Read the model definition and answer for the solid it produces. Units are mm, in the model's axes. A direction names the side the tool comes from. Coordinates: 2 decimals unless noted, no trailing zeros. Loops run counter-clockwise (first coordinate to the right, second up) from the corner with the lowest first, then second, coordinate; pieces in that order, holes last. Notation, with made-up numbers: (-33.5, -35) - (-21.5, -35) arc R30 cw to (-21.5, -8) - close; hole circle Ø1 at (-4.75, -17). An arc over 180 degrees is marked (long way). Use CSV: the item, a comma, the result in double quotes.
```python
from build123d import *

# Parameters (mm, degrees)
SKETCH1_R           = 30
BOSS_EXTRUDE1_DEPTH = 13
SKETCH2_R           = 32.5
BOSS_EXTRUDE2_DEPTH = 1
SKETCH3_R           = 1.6
CUT_EXTRUDE1_DEPTH  = 3.5
SKETCH4_R           = 14
CUT_EXTRUDE2_DEPTH  = 51
SKETCH5_R           = 2.6
CUT_EXTRUDE3_DEPTH  = 25


with BuildPart() as part:
    # Sketch1 → Boss-Extrude1 (new body)
    with BuildSketch(Plane(origin=(0, 0, 0), x_dir=(1, 0, 0), z_dir=(0, 1, 0))):
        with Locations(Location((0, 0, 0), (0, 0, 90))):
            Circle(SKETCH1_R)
    extrude(amount=BOSS_EXTRUDE1_DEPTH)

    # Sketch2 → Boss-Extrude2 (add)
    with BuildSketch(Plane.XZ):
        with Locations(Location((0, 0, 0), (0, 0, 270))):
            Circle(SKETCH2_R)
    extrude(amount=-BOSS_EXTRUDE2_DEPTH)

    # Sketch3 → Cut-Extrude1 (cut)
    with BuildSketch(Plane(origin=(0, 0, 0), x_dir=(1, 0, 0), z_dir=(0, 1, 0))):
        with Locations(Location((0, 25, 0), (0, 0, 270))):
            Circle(SKETCH3_R)
        with Locations(Location((21.650635095, 12.5, 0), (0, 0, 270))):
            Circle(SKETCH3_R)
        with Locations(Location((21.650635095, -12.5, 0), (0, 0, 270))):
            Circle(SKETCH3_R)
        with Locations(Location((0, -25, 0), (0, 0, 270))):
            Circle(SKETCH3_R)
        with Locations(Location((-21.650635095, -12.5, 0), (0, 0, 270))):
            Circle(SKETCH3_R)
        with Locations(Location((-21.650635095, 12.5, 0), (0, 0, 270))):
            Circle(SKETCH3_R)
    extrude(amount=CUT_EXTRUDE1_DEPTH, mode=Mode.SUBTRACT)

    # Sketch4 → Cut-Extrude2 (cut)
    with BuildSketch(Plane.XZ):
        with Locations(Location((0, 0, 0), (0, 0, 270))):
            Circle(SKETCH4_R)
    extrude(amount=-CUT_EXTRUDE2_DEPTH, mode=Mode.SUBTRACT)

    # Sketch5 → Cut-Extrude3 (cut)
    with BuildSketch(Plane.XZ):
        with Locations(Location((-12.5, 21.650635095, 0), (0, 0, 270))):
            Circle(SKETCH5_R)
        with Locations(Location((12.5, 21.650635095, 0), (0, 0, 270))):
            Circle(SKETCH5_R)
        with Locations(Location((25, 0, 0), (0, 0, 270))):
            Circle(SKETCH5_R)
        with Locations(Location((12.5, -21.650635095, 0), (0, 0, 270))):
            Circle(SKETCH5_R)
        with Locations(Location((-12.5, -21.650635095, 0), (0, 0, 270))):
            Circle(SKETCH5_R)
        with Locations(Location((-25, 0, 0), (0, 0, 270))):
            Circle(SKETCH5_R)
    extrude(amount=-CUT_EXTRUDE3_DEPTH, mode=Mode.SUBTRACT)


solid = part.part
```
Q1. The part is cut by section C-C on x = -2.5. Determine the outline of the cut face in (y, z).
Reported:
outline,"(0, -32.4) - (1, -32.4) - (1, -29.9) - (13, -29.9) - (13, -13.77) - (0, -13.77) - close; (0, 13.77) - (13, 13.77) - (13, 29.9) - (1, 29.9) - (1, 32.4) - (0, 32.4) - close"
Q2. The part is cut by section D-D on y = 1.75. Give the number of separate pieces and of enclosed holes in the cut face, and give its area (3 significant figures).
Reported:
separate pieces,"1"
enclosed holes,"13"
area,"2,040 mm²"
Q3. Given P1, Ø4, axis at x = 25, z = 0, coming from the +Y side; P2, Ø1.6, axis at x = 21, z = 12.5, coming from the -Y side; P3, Ø1.5, axis at y = 10.5, z = -11.5, coming from the -X side; P4, Ø4, axis at x = 9.5, y = 5, coming from the -Z side, each flat-ended and moving along its own axis, determine where each tip first touches the part or whether it passes through.
Reported:
P1,"passes through"
P2,"stops at y = 3.5"
P3,"stops at x = -28.01"
P4,"stops at z = -29.05"
Q4. The part is cut by section B-B on z = -22. Determine the outline of the cut face in (x, y), and give its area (3 significant figures).
Reported:
outline,"(-23.92, 0) - (-15.08, 0) - (-15.08, 13) - (-20.4, 13) - (-20.4, 1) - (-23.92, 1) - close; (-9.92, 0) - (9.92, 0) - (9.92, 13) - (-9.92, 13) - close; (15.08, 0) - (23.92, 0) - (23.92, 1) - (20.4, 1) - (20.4, 13) - (15.08, 13) - close"
area,"403 mm²"
Q5. A tool of negligible diameter and unlimited length cuts with its end or side. For faces 4 (the face through (9.96, 6.41, -21.09)), 5 (the face through (22, 3.5, -13)), 6 (the face through (-29, 1, -9)), from which of +Z, -Z, +X, -X, +Y, -Y can it reach the whole face along a straight path? Write none if from no direction.
Reported:
face 4,"+Y, -Y"
face 5,"-Y"
face 6,"+Y"
Q6. The part is cut by section A-A on y = 6.75. Determine the outline of the cut face in (x, z).
Reported:
outline,"circle Ø60 at (0, 0); hole circle Ø5.2 at (-25, 0); hole circle Ø5.2 at (-12.5, -21.65); hole circle Ø5.2 at (-12.5, 21.65); hole circle Ø28 at (0, 0); hole circle Ø5.2 at (12.5, -21.65); hole circle Ø5.2 at (12.5, 21.65); hole circle Ø5.2 at (25, 0)"
Q7. For a pull along Z with two mould halves and no side action, classify faces 1 (the face through (0, 0, 15)), 2 (the face through (-13.67, 6.41, 3.03)), 3 (the face through (9.76, 0.49, -31)) as +Z half, -Z half, draft (parallel to the pull), parting line (faces both ways), or undercut.
Reported:
face 1,"draft"
face 2,"undercut"
face 3,"parting line"
Q8. Find the intervals of material crossed by probe 1 along Z at (x, y) = (-10.5, 2); probe 2 along X at (y, z) = (12.5, 22); probe 3 along X at (y, z) = (9, -21), in increasing order. Write a range as [from, to].
Reported:
probe 1,"z = [-28.1, -23.31], [-19.99, -9.26], [9.26, 19.99], [23.31, 28.1]"
probe 2,"x = [-20.4, -15.08], [-9.92, 9.92], [15.08, 20.4]"
probe 3,"x = [-21.42, -15.02], [-9.98, 9.98], [15.02, 21.42]"
